Design review of the part built by this model. Coordinates are the model's own, in mm. A direction names the side the tool comes from. Round coordinates to 2 decimals unless told otherwise and drop trailing zeros. Order: outer loops, then holes, each group sorted by start corner. A loop starts at its lowest first (then second) coordinate and runs counter-clockwise, first axis right, second up. Notation, with made-up numbers: (82.5, 5.5) - (118.5, 5.5) arc R26 cw to (118.5, 41.5) - close; hole circle Ø11 at (47, -36). An arc over 180 degrees is marked (long way). Write item = value, one per line.
from build123d import *

# Parameters (mm, degrees)
F3_R = 5.08
F4_R = 25.4
F5_R = 2.54


with BuildPart() as f2:
    # F0 (on Front) → F2 (revolve)
    with BuildSketch(Plane.XZ):
        Polygon((52.705, 6.35), (52.705, 0), (56.515, 0), (56.515, 6.35), (10.16, 76.2), (10.16, 88.9), (6.35, 88.9), (6.35, 76.2), align=None)
    revolve(axis=Axis((0, 0, 41.439734), (0, 0, -1)))

    # F3
    f3_edges = [f2.edges().sort_by_distance(p)[0] for p in [
        (-10.16, 0, 76.2),
    ]]
    fillet(f3_edges, radius=F3_R)

    # F4
    f4_edges = [f2.edges().sort_by_distance(p)[0] for p in [
        (-6.35, 0, 76.2),
    ]]
    fillet(f4_edges, radius=F4_R)

    # F5
    f5_edges = [f2.edges().sort_by_distance(p)[0] for p in [
        (-6.35, 0, 88.9),
    ]]
    fillet(f5_edges, radius=F5_R)


solid = f2.part
1) We need section A-A on z = 63. Write out the cut boundary in (x, y).
Findings:
outline = circle Ø37.84 at (0, 0); hole circle Ø30.22 at (0, 0)
2) For faces 1 (the cylindrical face through (-1.323, -10.074, 83.394)), 2 (the cylindrical face through (-11.43, 51.45, 3.13)), 3 (the cylindrical face through (6.057, -1.907, 85.093)), list the 3-axis set-ups (+Z, -Z, +X, -X, +Y, -Y) from which the entire face can be reached by the end or side of a thin tool; tool diameter is ignored.
Findings:
face_1 = +Z
face_2 = -Z
face_3 = +Z, -Z
3) We need section B-B on z = 33.5. Write out the cut boundary in (x, y).
Findings:
outline = circle Ø76.99 at (0, 0); hole circle Ø69.37 at (0, 0)
4) The part is to be moulded in two halves that separate along Y. For faces 4 (the conical face through (-4.895, 22.044, 51.743)), 5 (the conical face through (22.25, -7.01, 56.36)), 6 (the flat face through (1, 9, 88.9)), say which applies: released by +Y, released by -Y, zero draft, split by the parting line, or undercut.
Findings:
face_4 = undercut
face_5 = split by the parting line
face_6 = zero draft
5) Clearance check with flat-ended pins moving along their axes: pin 1 Ø5 at (x, z) = (11, 57) entering from +Y; pin 2 Ø1.5 at (x, y) = (36.5, -0.5) entering from -Z; pin 3 Ø1.5 at (x, z) = (-25, 58.5) entering from -Y; pin 4 Ø10 at (x, z) = (-9, 55) entering from +Y. State where each tip first meets the part, or that it passes through.
Findings:
pin_1 = 22.3
pin_2 = 29.63
pin_3 = through
pin_4 = 26.36
6) To check wall thickness, follow L1, parallel to X at y = 0, z = 85; L2, parallel to Y at x = 0, z = 4 (3 decimals). State the ranges of each line that lie inside material, in increasing order. Write a range as from..to.
Findings:
L1 = -10.16..-6.35, 6.35..10.16
L2 = -56.515..-52.705, 52.705..56.515
